Design review of the part built by this model. Coordinates are the model's own, in mm. Round coordinates to 2 decimals unless told otherwise and drop trailing zeros. Order: outer loops, then holes, each group sorted by start corner. A loop starts at its lowest first (then second) coordinate and runs counter-clockwise, first axis right, second up.
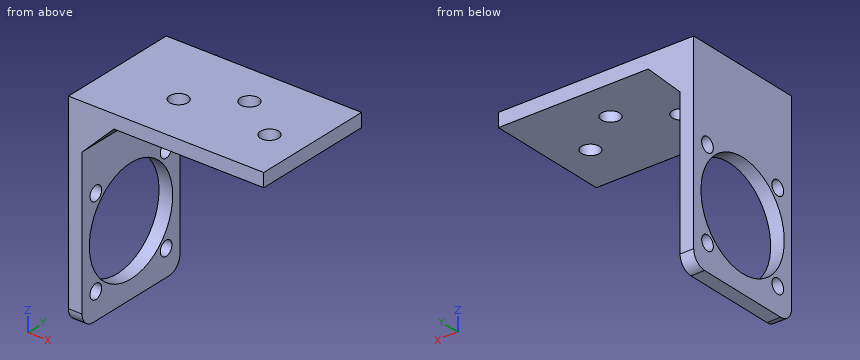
from build123d import *

# Parameters (mm, degrees)
SKETCH005_W             = 27
SKETCH005_H             = 40
SKETCH005_R             = 2
PAD003_DEPTH            = 3
SKETCH004_R             = 11.5
SKETCH004_R_2           = 1.6
PAD004_DEPTH            = 3
PAD024_DEPTH            = 27
BODY002_ROLL_ANGLE      = -89.9826768737
BODY002_PITCH_ANGLE     = -0.0173178896
BODY002_PLACEMENT_ANGLE = 89.9826768737


with BuildPart() as part:
    # Sketch005 → Pad003 (new body)
    with BuildSketch(Plane.XZ):
        with Locations((13.5, -20)):
            Rectangle(SKETCH005_W, SKETCH005_H)
        with Locations((11, -12.5)):
            Circle(SKETCH005_R, mode=Mode.SUBTRACT)
        with Locations((18, -22.5)):
            Circle(SKETCH005_R, mode=Mode.SUBTRACT)
        with Locations((11, -32.5)):
            Circle(SKETCH005_R, mode=Mode.SUBTRACT)
    extrude(amount=-PAD003_DEPTH)

    # Sketch004 → Pad004 (join)
    with BuildSketch(Plane.XY):
        with BuildLine():
            Line((0, 42), (0, 0))
            Line((0, 0), (27, 0))
            Line((27, 0), (27, 42))
            ThreePointArc((27, 42), (26.1213203436, 44.1213203436), (24, 45))
            Line((24, 45), (3, 45))
            ThreePointArc((3, 45), (0.8786796564, 44.1213203436), (0, 42))
        make_face()
        with Locations((13.5, 29.5)):
            Circle(SKETCH004_R, mode=Mode.SUBTRACT)
        with Locations((3.8, 39.2)):
            Circle(SKETCH004_R_2, mode=Mode.SUBTRACT)
        with Locations((23.2, 39.2)):
            Circle(SKETCH004_R_2, mode=Mode.SUBTRACT)
        with Locations((23.2, 19.8)):
            Circle(SKETCH004_R_2, mode=Mode.SUBTRACT)
        with Locations((3.8, 19.8)):
            Circle(SKETCH004_R_2, mode=Mode.SUBTRACT)
    extrude(amount=PAD004_DEPTH)

    # Sketch043 → Pad024 (join)
    with BuildSketch(Plane.YZ):
        Polygon((0, 0), (0, -10), (10, 0), align=None)
    extrude(amount=PAD024_DEPTH)


with BuildPart() as part_1:
    # Body002 roll: moved
    add(part.part.rotate(Axis((0, 0, 0), (1, 0, 0)), BODY002_ROLL_ANGLE))


with BuildPart() as part_2:
    # Body002 pitch: moved
    add(part_1.part.rotate(Axis((0, 0, 0), (0, 1, 0)), BODY002_PITCH_ANGLE))


with BuildPart() as part_3:
    # Body002 placement: moved
    add(part_2.part.moved(Location((-70, 7, 0))).rotate(Axis((-70, 7, 0), (0, 0, 1)), BODY002_PLACEMENT_ANGLE))


solid = part_3.part
1) Take a section at A-A on y = 30.25. State how many separate pieces and enclosed holes the cut face has, plus the area to 3 significant figures.
Results:
separate pieces: 4
enclosed holes: 0
area: 224 mm2
2) Clearance check with flat-ended pins moving along their axes: P1, Ø4, axis at y = 26, z = -4.5, coming from the -X side; P2, Ø8, axis at x = -35, y = 12, coming from the -Z side; P3, Ø3.5, axis at y = 15.5, z = -1.5, coming from the +X side. State where each tip first meets the part, or that it passes through.
Results:
P1: stops at x = -73
P2: stops at z = -3.01
P3: stops at x = -30
3) Take a section at B-B on x = -41.5. Give the boundary of the cut face in (y, z), plus the area to 3 significant figures.
Results:
outline: (6.99, -3.01) - (33.99, -3) - (33.99, 0) - (6.99, -0.01) - close
area: 81.0 mm2
4) To check wall thickness, follow line 1 along Y through (x, z) = (-51, -1.5); line 2 along X through (y, z) = (8, -14); line 3 along Z through (x, y) = (-49.5, 22.5). State the ranges of each line that lie inside material, in increasing order.
Results:
line 1: y = 6.99 to 33.99
line 2: x = -73 to -70
line 3: z = -3 to 0
5) Take a section at C-C on z = -17. Give the boundary of the cut face in (x, y), plus the area to 3 significant figures.
Results:
outline: (-73.01, 7.01) - (-70.01, 7.01) - (-70, 34.01) - (-73, 34.01) - close
area: 81.0 mm2
